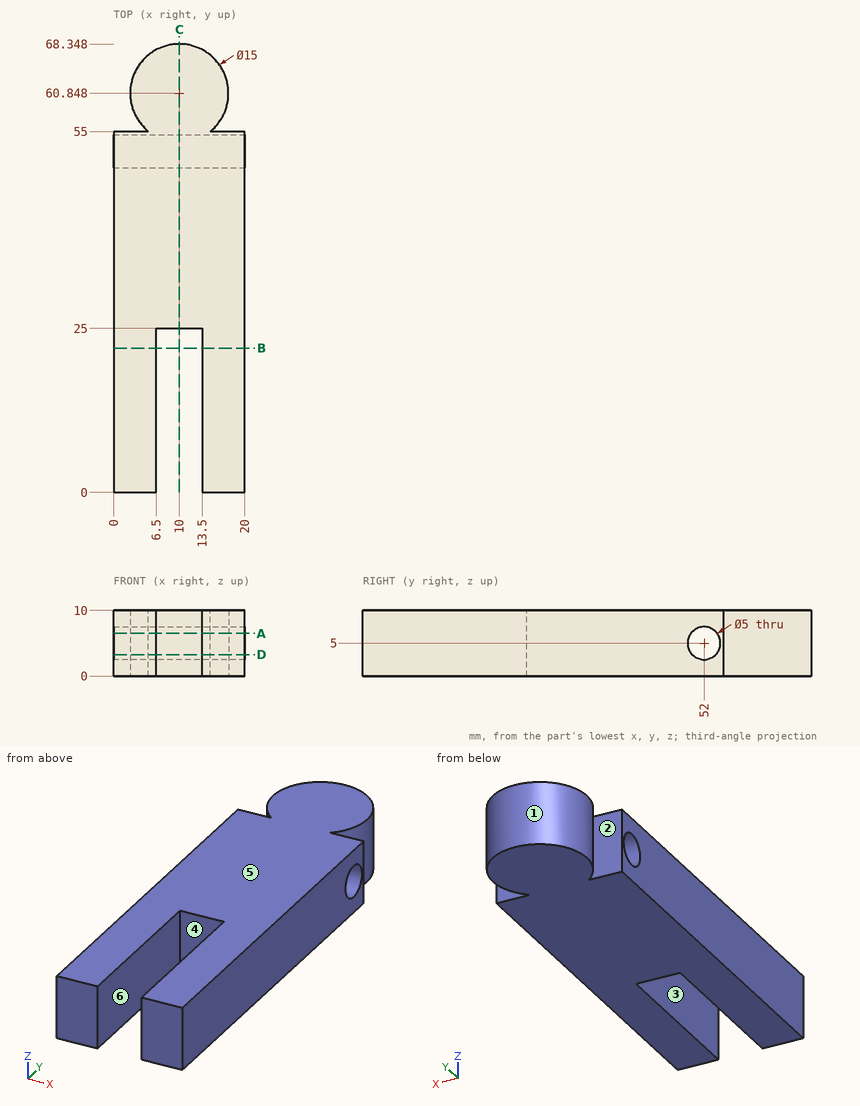
The figure shows three views and two pictorial views of one solid part (mm, origin at its lowest corner). Answer the questions. A direction names the side the tool comes from. Round coordinates to 2 decimals unless told otherwise and drop trailing zeros. Order: outer loops, then holes, each group sorted by start corner. A loop starts at its lowest first (then second) coordinate and runs counter-clockwise, first axis right, second up. Notation, with made-up numbers: (77, -24) -> (109, -24) arc R21 cw to (109, 6) -> close; hole circle Ø3 at (20, -28.5). An arc over 180 degrees is marked (long way). Put each result on its own line as item: value.
Q1. Which of the six approach directions +Z, -Z, +X, -X, +Y, -Y give full straight-line access (tool end or side, diameter ignored) to the marked faces 5 and 6?
Results list:
face 5: +Z, +X, -X, +Y, -Y
face 6: +Z, -Z, -Y
Q2. Section B-B, the plane y = 22 is taken. Write down the section's boundary in (x, z), and give its area (3 significant figures).
Results list:
outline: (0, 0) -> (6.5, 0) -> (6.5, 10) -> (0, 10) -> close; (13.5, 0) -> (20, 0) -> (20, 10) -> (13.5, 10) -> close
area: 130 mm^2
Q3. Section A-A, the plane z = 6.5 is taken. Write down the section's boundary in (x, y) (1 decimal).
Results list:
outline: (0, 0) -> (6.5, 0) -> (6.5, 25) -> (13.5, 25) -> (13.5, 0) -> (20, 0) -> (20, 50) -> (0, 50) -> close; (0, 54) -> (20, 54) -> (20, 55) -> (14.7, 55) arc R7.5 ccw (long way) to (5.3, 55) -> (0, 55) -> close
Q4. Section D-D, the plane z = 3.25 is taken. Write down the section's boundary in (x, y) (1 decimal).
Results list:
outline: (0, 0) -> (6.5, 0) -> (6.5, 25) -> (13.5, 25) -> (13.5, 0) -> (20, 0) -> (20, 50.2) -> (0, 50.2) -> close; (0, 53.8) -> (20, 53.8) -> (20, 55) -> (14.7, 55) arc R7.5 ccw (long way) to (5.3, 55) -> (0, 55) -> close
Q5. Section C-C, the plane x = 10 is taken. Write down the section's boundary in (y, z).
Results list:
outline: (25, 0) -> (68.35, 0) -> (68.35, 10) -> (25, 10) -> close; hole circle Ø5 at (52, 5)
Q6. Each of these flat-tipped pins is pushed along its axis until it touches: P1, Ø3.5, axis at x = 9, z = 6.5, coming from the -Y side; P2, Ø4, axis at x = 17.5, z = 4, coming from the +Y side; P3, Ø4, axis at x = 2, z = 3, coming from the +Y side. Where does it stop, or does it pass through?
Results list:
P1: y = 25
P2: y = 65.95
P3: y = 65.35
Q7. Determine the mould class of the marked faces 1, 2, 3 and 4 for opening direction Y: pulls with the +Y half, pulls with the -Y half, needs draft (parallel to the pull), parting line crosses it, or undercut.
Results list:
face 1: undercut
face 2: undercut
face 3: needs draft
face 4: pulls with the -Y half
Q8. Consider line 1 along X through (y, z) = (12.5, 2.25); line 2 along Y through (x, z) = (13, 5); line 3 along Y through (x, z) = (1.5, 6.75) (1 decimal). Determine where each line is inside the solid, lowest interval first.
Results list:
line 1: 0 to 6.5, 13.5 to 20
line 2: 25 to 49.5, 54.5 to 67.72
line 3: 0 to 50.2, 53.8 to 55
